Autodesk Inventor part; units mm, degrees
ref_plane "to_housing_XY" through (0, 0, 0) normal (1, 0, 0) x (0, 0, -1)
ref_plane "to_housing_YZ" through (0, 0, 0) normal (0, 0, -1) x (0, 1, 0)
ref_plane "to_housing_ZX" through (0, 0, 0) normal (0, 1, 0) x (1, 0, 0)
sketch "Sketch_1" plane through (0, 0, 0) normal (0, 0, 1) x (1, 0, 0)
  line L0 (2.9, 0) -> (0.1, 0)
  arc A0 (0, 3.1) -> (0.1, 3) centre (0.1, 3.1) ccw
  line L1 (0.1, 3) -> (2.9, 3)
  arc A1 (2.9, 3) -> (3, 3.1) centre (2.9, 3.1) ccw
  line L2 (3, 3.1) -> (3, 3.55)
  line L3 (3, 3.55) -> (2.73, 3.55)
  line L4 (2.73, 3.55) -> (2.73, 4.6)
  line L5 (2.73, 4.6) -> (3, 4.6)
  line L6 (3, 4.6) -> (3, 4.9)
  arc A2 (3, 4.9) -> (2.9, 5) centre (2.9, 4.9) ccw
  line L7 (2.9, 5) -> (0.1, 5)
  arc A3 (0.1, 5) -> (0, 4.9) centre (0.1, 4.9) ccw
  line L8 (0, 4.9) -> (0, 4.6)
  line L9 (0, 4.6) -> (0.27, 4.6)
  line L10 (0.27, 4.6) -> (0.27, 3.55)
  line L11 (0.27, 3.55) -> (0, 3.55)
  line L12 (0, 3.55) -> (0, 3.1)
revolve "Revolution1" add sketch "Sketch_1" angle 360 about axis through (2.9, 0, 0) along (1, 0, 0)
ref_plane "to_housing_XY" through (0, 0, 0) normal (1, 0, 0) x (0, 0, -1)
ref_plane "to_housing_YZ" through (0, 0, 0) normal (0, 0, -1) x (0, 1, 0)
ref_plane "to_housing_ZX" through (0, 0, 0) normal (0, 1, 0) x (1, 0, 0)
ref_plane "to_housing_center_XY" through (1.5, 0, 0) normal (1, 0, 0) x (0, 0, -1)
ref_plane "to_housing_center_YZ" through (1.5, 0, 0) normal (0, 0, -1) x (0, 1, 0)
ref_plane "to_housing_center_ZX" through (1.5, 0, 0) normal (0, 1, 0) x (1, 0, 0)
properties part number "C-SE676ZZ"
Input: part model. Units: mm. Frame: model coordinates. A direction names the side the tool comes from. Coordinates: 2 decimals unless noted, no trailing zeros. Write each loop counter-clockwise with the first axis right and the second up, starting at its lowest first coordinate (ties: lowest second). Pieces come first, ordered by that corner, then holes. Notation, with made-up numbers: M 42.5,1 L 63.5,1 A13 ccw 63.5,20 Z; hole C 0,56 d8. An arc over 180 degrees is marked long. Answer as a JSON object with one key per item and string values. Group by question number.
(1) Section C-C on x = 1.35. Output: boundary loops of the cut face in (y, z), plus the area to 3 significant figures.
(2) Ray query, line 1 along Z through (x, y) = (2.9, 0); line 2 along Z through (x, y) = (2.8, -1.25); line 3 along Z through (x, y) = (1.05, 0). Return the intervals inside material, ascending. Write a range as [from, to].
(3) Contact query for flat-ended pins moving along their axis: P1, Ø1.5, axis at x = 1, y = 2, coming from the -Z side; P2, Ø5.5, axis at y = 0, z = 0, coming from the +X side. Output: stop coordinate, or through.
(4) Set-up query: faces 3 (the face through (2.73, 0, -4)), 4 (the face through (2, -3, 0)). Return all of +Z, -Z, +X, -X, +Y, -Y with unobstructed straight access to the full face (end or side cutting, diameter ignored); none if empty.
(5) Mould query, pull axis Y, two halves, no side actions, for faces 1 (the face through (1.48, -1.08, 4.88)), 2 (the face through (0.27, 0, -4)). Classes: pulls with the +Y half, pulls with the -Y half, needs draft (parallel to the pull), parting line crosses it, or undercut.
Result set:
{
 "1": {"outline": "C 0,0 d10; hole C 0,0 d6", "area": "50.3 mm2"},
 "2": {"line 1": "z = [-5, -4.6], [-3.55, -3], [3, 3.55], [4.6, 5]", "line 2": "z = [-4.84, -4.43], [-3.32, -2.73], [2.73, 3.32], [4.43, 4.84]", "line 3": "z = [-5, -3], [3, 5]"},
 "3": {"P1": "stops at z = -4.84", "P2": "passes through"},
 "4": {"face 3": "+X", "face 4": "+X, -X"},
 "5": {"face 1": "parting line crosses it", "face 2": "undercut"}
}
